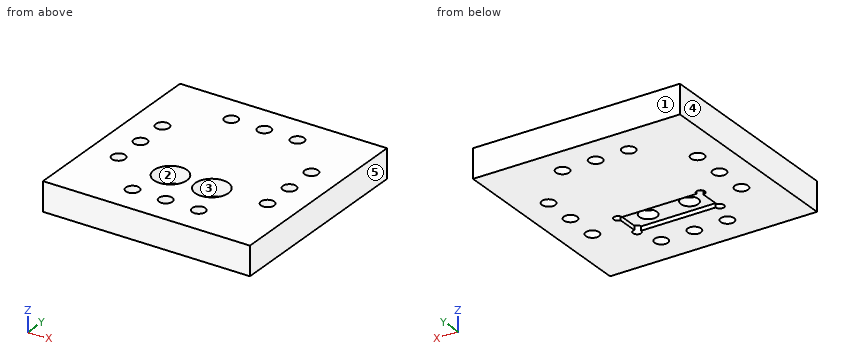
```python
from build123d import *

# Parameters (mm, degrees)
F0_W           = 50
F0_H           = 50
F1_DEPTH       = 7
F3_D           = 3.2
F4_D           = 4.2
F4_CBORE_D     = 8
F4_CBORE_DEPTH = 4
F5_W           = 20
F5_H           = 7
F5_R           = 2.1
F6_DEPTH       = 1
F7_D           = 2
F7_DEPTH       = 1
F7_START       = 1
F7_TIP         = 0.600860619


with BuildPart() as f1:
    # F0 (on Top) → F1 (new body)
    with BuildSketch(Plane.XY):
        Rectangle(F0_W, F0_H)
    extrude(amount=F1_DEPTH)

    # F3 (through all)
    with Locations(Plane.XY.offset(7)):
        with Locations((-18, 8), (-18, 0), (-18, -8), (-8, -18), (0, -18), (8, -18), (18, -8), (18, 0), (18, 8), (-8, 18), (0, 18), (8, 18)):
            Hole(F3_D / 2)

    # F4 (through all)
    with Locations(Plane.XY.offset(7)):
        with Locations((-5, -8.7), (5, -8.7)):
            CounterBoreHole(F4_D / 2, F4_CBORE_D / 2, F4_CBORE_DEPTH)

    # F5 (on face) → F6 (cut)
    with BuildSketch(Plane(origin=(0, 0, 0), x_dir=(1, 0, 0), z_dir=(0, 0, -1))):
        with Locations((0, 8.7)):
            Rectangle(F5_W, F5_H)
        with Locations((-5, 8.7)):
            Circle(F5_R, mode=Mode.SUBTRACT)
        with Locations((5, 8.7)):
            Circle(F5_R, mode=Mode.SUBTRACT)
    extrude(amount=-F6_DEPTH, mode=Mode.SUBTRACT)

    # F7
    # its depths count from where the whole tool has entered the part; down to there all is cleared
    with Locations(Plane(origin=(0, 0, 0), x_dir=(1, 0, 0), z_dir=(0, 0, -1)).offset(-F7_START)):
        with Locations((-10, 5.2), (-10, 12.2), (10, 12.2), (10, 5.2)):
            Hole(F7_D / 2, depth=F7_DEPTH)
            with Locations((0, 0, -(F7_DEPTH + F7_TIP / 2))):  # 118° drill point
                Cone(0, F7_D / 2, F7_TIP, mode=Mode.SUBTRACT)


solid = f1.part
```
The model under review builds one solid part; all positions refer to its coordinate system, in mm. Face numbers are marked on the shaded views. A direction names the side the tool comes from. Round coordinates to 2 decimals unless told otherwise and drop trailing zeros. Loops run counter-clockwise (first coordinate to the right, second up) from the corner with the lowest first, then second, coordinate; pieces in that order, holes last. Notation, with made-up numbers: (-23.5, 58) - (32.5, 58) arc R12 ccw to (32.5, 77) - close; hole circle Ø7 at (-9, 44). An arc over 180 degrees is marked (long way). Use a Markdown table: item, result. Add a question column.
Q1. Insertion check: pin 1 Ø4 at (x, y) = (0, 18) entering from -Z; pin 2 Ø1.5 at (x, y) = (7, -10) entering from -Z; pin 3 Ø1.9 at (x, y) = (8, 18) entering from +Z; pin 4 Ø1.6 at (x, y) = (-10, -12.2) entering from -Z. Each pin has a flat end and moves straight along its axis. Give the tip position at first contact, or say it passes through.
Q2. Add section D-D (y = -18). State the section outline as (x, z) points.
Q3. Add section A-A (y = 0). State the section outline as (x, z) points, plus the area to 3 significant figures.
Q4. Add section B-B (x = 0). State the section outline as (y, z) points.
Q5. The part is to be moulded in two halves that separate along X. For the marked faces 3, 4 and 5, say which applies: pulls with the +X half, pulls with the -X half, needs draft (parallel to the pull), parting line crosses it, or undercut.
Q6. For probe 1 along Y at (x, z) = (-8, 2); probe 2 along Y at (x, z) = (8, 0.75); probe 3 along X at (y, z) = (1, 0.5), list the stretches that pass through material, from the lowest coordinate up.
Q7. Add section C-C (z = 5.5). State how many separate pieces and enclosed holes the cut face has, plus the area to 3 significant figures.
Q8. Machinability: for the marked faces 1 and 2, which of the approach directions +Z, -Z, +X, -X, +Y, -Y give a long, thin tool a straight path to every point of the face, cutting with its end or side? Answer none if there is none.
Worked answers:
| question | item | result |
|---|---|---|
| 1 | pin 1 | z = 0 |
| 1 | pin 2 | z = 1 |
| 1 | pin 3 | through |
| 1 | pin 4 | z = 2.12 |
| 2 | outline | (-25, 0) - (-9.6, 0) - (-9.6, 7) - (-25, 7) - close; (-6.4, 0) - (-1.6, 0) - (-1.6, 7) - (-6.4, 7) - close; (1.6, 0) - (6.4, 0) - (6.4, 7) - (1.6, 7) - close; (9.6, 0) - (25, 0) - (25, 7) - (9.6, 7) - close |
| 3 | outline | (-25, 0) - (-19.6, 0) - (-19.6, 7) - (-25, 7) - close; (-16.4, 0) - (16.4, 0) - (16.4, 7) - (-16.4, 7) - close; (19.6, 0) - (25, 0) - (25, 7) - (19.6, 7) - close |
| 3 | area | 305 mm² |
| 4 | outline | (-25, 0) - (-19.6, 0) - (-19.6, 7) - (-25, 7) - close; (-16.4, 0) - (-12.2, 0) - (-12.2, 1) - (-5.2, 1) - (-5.2, 0) - (16.4, 0) - (16.4, 7) - (-16.4, 7) - close; (19.6, 0) - (25, 0) - (25, 7) - (19.6, 7) - close |
| 5 | face 3 | undercut |
| 5 | face 4 | pulls with the -X half |
| 5 | face 5 | pulls with the +X half |
| 6 | probe 1 | -25 to -19.6, -16.4 to 16.4, 19.6 to 25 |
| 6 | probe 2 | -25 to -19.6, -16.4 to -12.2, -5.2 to 16.4, 19.6 to 25 |
| 6 | probe 3 | -25 to -19.25, -16.75 to 16.75, 19.25 to 25 |
| 7 | separate pieces | 1 |
| 7 | enclosed holes | 14 |
| 7 | area | 2,300 mm² |
| 8 | face 1 | +Z, -Z, +X, -X, +Y |
| 8 | face 2 | +Z |
